Verification items for the finished model (mm, model axes). Face numbers are marked on the shaded views. A direction names the side the tool comes from. Coordinates: 2 decimals unless noted, no trailing zeros. Write each loop counter-clockwise with the first axis right and the second up, starting at its lowest first coordinate (ties: lowest second). Pieces come first, ordered by that corner, then holes. Notation, with made-up numbers: M 22,-33 L 59,-33 A32 cw 59,-2 Z; hole C 65.5,39 d2. An arc over 180 degrees is marked long. Answer in a Markdown table with one row per item.
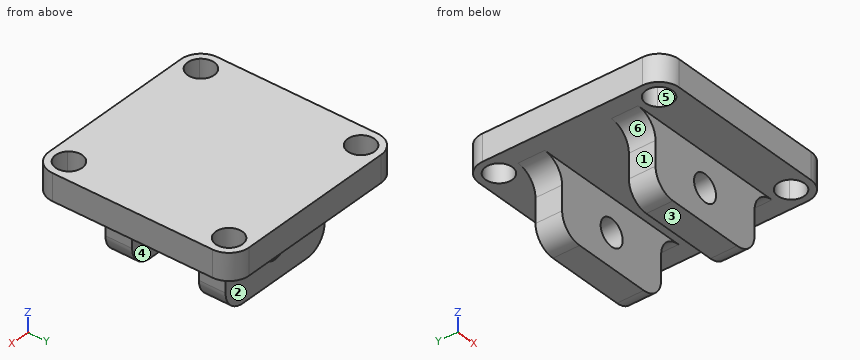
Autodesk Inventor part; units mm, degrees
ref_plane "YZ Plane" through (0, 0, 0) normal (1, 0, 0) x (0, 1, 0)
ref_plane "XZ Plane" through (0, 0, 0) normal (0, 1, 0) x (-1, 0, 0)
ref_plane "XY Plane" through (0, 0, 0) normal (0, 0, 1) x (1, 0, 0)
ref_plane "Work Plane1" through (-192, 24, -212) normal (0, 0, -1) x (-1, 0, 0)
sketch "Sketch1" plane through (-192, 24, -212) normal (0, 0, -1) x (-1, 0, 0)
  circle A0 centre (-32, -8) radius 2
  arc A1 (-30.5858, -33.4142) -> (-33.4142, -30.5858) centre (-32, -32) ccw
  arc A2 (-6.5858, -33.4142) -> (-9.4142, -30.5858) centre (-8, -32) ccw
  circle A3 centre (-8, -8) radius 2
  circle A4 centre (-32, -32) radius 2
  circle A5 centre (-8, -32) radius 2
  circle A6 centre (-8, -8) radius 2
  circle A7 centre (-32, -8) radius 2
  circle A8 centre (-32, -8) radius 3
  circle A9 centre (-8, -8) radius 3
  circle A10 centre (-8, -32) radius 3
  circle A11 centre (-32, -32) radius 3
  line L0 (-35, -8) -> (-35, -32)
  line L1 (-32, -35) -> (-8, -35)
  line L2 (-5, -32) -> (-5, -8)
  line L3 (-8, -5) -> (-32, -5)
  point P0 (-192, -24)
  point P1 (-9.4142, -30.5858)
  point P2 (-33.4142, -30.5858)
  dimension "d0" = 1
  dimension "d1" = 1
  dimension "d2" = 1
  dimension "d3" = 1
extrude "Extrusion1" add sketch "Sketch1" along normal blind 4
sketch "Sketch2" plane through (-192, 24, -216) normal (0, 0, -1) x (-1, 0, 0)
  line L0 (-35, -8) -> (-35, -32)
  line L1 (-5, -32) -> (-5, -8)
  line L2 (-5, -32) -> (-5, -8)
  line L3 (-35, -11) -> (-5, -11)
  line L4 (-5, -11) -> (-5, -29)
  line L5 (-5, -29) -> (-35, -29)
  line L6 (-35, -29) -> (-35, -11)
  circle A0 centre (-32, -8) radius 2
  circle A1 centre (-8, -8) radius 2
  circle A2 centre (-8, -32) radius 2
  circle A3 centre (-32, -32) radius 2
  line L7 (-29, -11) -> (-29, -29)
  line L8 (-11, -11) -> (-11, -29)
  point P0 (-192, -24)
  dimension "d6" = 3
  dimension "d7" = 3
  dimension "d8" = 3
  dimension "d9" = 3
extrude "Extrusion2" add sketch "Sketch2" along normal blind 10 contours L3 L8 L5 L7
sketch "Sketch3" plane through (-181, -5, -216) normal (-1, 0, 0) x (0, 0, 1)
  line L0 (0, 18) -> (0, 0)
  line L1 (0, 18) -> (-10, 18)
  line L2 (-10, 0) -> (-10, 18)
  line L3 (0, 0) -> (-10, 0)
  line L4 (-10, 18) -> (-10, 0)
  line L5 (0, 21) -> (0, -3)
  line L6 (-10, 14) -> (0, 14)
  line L7 (0, 14) -> (0, 4)
  line L8 (0, 4) -> (-10, 4)
  line L9 (-10, 4) -> (-10, 14)
  point P0 (216, 5)
  point P1 (-10, 4)
  point P2 (0, 4)
  point P3 (0, 14)
  dimension "d12" = 4
  dimension "d13" = 4
extrude "Extrusion3" cut sketch "Sketch3" against normal through all contours L0 L8 L2 L6
fillet "Fillet1" radius 3.175 8 edges at (-181, 11, -226) (-163, 11, -226) (-181, 11, -216) (-163, 11, -216) (-163, -3, -216) (-163, -3, -226) (-181, -3, -226) (-181, -3, -216)
sketch "Sketch4" plane through (-184.175, 13, -216) normal (0, 1, 0) x (1, 0, 0)
  arc A0 (21.175, 6.825) -> (18, 10) centre (18, 6.825) ccw
  line L0 (6.35, 10) -> (18, 10)
  arc A1 (6.35, 10) -> (3.175, 6.825) centre (6.35, 6.825) ccw
  line L1 (3.175, 3.175) -> (3.175, 6.825)
  arc A2 (0, 0) -> (3.175, 3.175) centre (0, 3.175) ccw
  line L2 (24.35, 0) -> (0, 0)
  arc A3 (21.175, 3.175) -> (24.35, 0) centre (24.35, 3.175) ccw
  line L3 (21.175, 3.175) -> (21.175, 6.825)
  circle A4 centre (12.175, 5) radius 2
  point P0 (184.175, -216)
  dimension "d17" = 4
  dimension "d18" = 18
  dimension "d19" = 9
  dimension "d20" = 10
  dimension "d21" = 5
extrude "Extrusion4" cut sketch "Sketch4" against normal through all contours A4
equation "\"d19\" = 0.5 * d18"
equation "\"d21\" = 0.5 * d20"
properties part number "hinge"
1) Sectioned sample at C-C (z = -224.25). Record the cut outline in (x, y), then the cut area to 3 significant figures.
Response values:
| item | result |
|---|---|
| outline | M -180.66,-5 L -163.34,-5 L -163.34,-1 L -180.66,-1 Z; M -180.66,9 L -163.34,9 L -163.34,13 L -180.66,13 Z |
| area | 139 mm² |
2) Tool access check on the marked faces 1, 2 and 3. Record the directions out of +Z, -Z, +X, -X, +Y, -Y that give a thin tool (end or side, any length) a straight path to the whole face; none if there is none.
Response values:
| item | result |
|---|---|
| face 1 | -Z, -X, +Y, -Y |
| face 2 | -Z, +X, -X, +Y |
| face 3 | -Z, +X, -X, +Y, -Y |
3) Release check for a two-part mould opening along X. For the marked faces 4, 5 and 6 record: +X half, -X half, draft (parallel to the pull), parting line (faces both ways), or undercut.
Response values:
| item | result |
|---|---|
| face 4 | draft |
| face 5 | undercut |
| face 6 | -X half |
4) Sectioned sample at B-B (y = -3.5). Record the cut outline in (x, z) (3 decimals).
Response values:
| item | result |
|---|---|
| outline | M -187,-216 L -184.175,-216 A3.175 cw -181,-219.175 L -181,-222.825 A3.175 ccw -177.825,-226 L -166.175,-226 A3.175 ccw -163,-222.825 L -163,-219.175 A3.175 cw -159.825,-216 L -157,-216 L -157,-212 L -187,-212 Z; hole C -172,-221 d4 |
5) Sectioned sample at D-D (z = -221.5). Record the cut outline in (x, y), then the cut area to 3 significant figures.
Response values:
| item | result |
|---|---|
| outline | M -181,-5 L -173.94,-5 L -173.94,-1 L -181,-1 Z; M -181,9 L -173.94,9 L -173.94,13 L -181,13 Z; M -170.06,-5 L -163,-5 L -163,-1 L -170.06,-1 Z; M -170.06,9 L -163,9 L -163,13 L -170.06,13 Z |
| area | 113 mm² |
6) Thickness scan on L1, parallel to Y at x = -184, z = -214.4; L2, parallel to Y at x = -169, z = -217; L3, parallel to Z at x = -172, y = -1.9. Record the ranges inside material, lowest first. Write a range as [from, to].
Response values:
| item | result |
|---|---|
| L1 | y = [-11, -10], [-6, 14], [18, 19] |
| L2 | y = [-5, -1], [9, 13] |
| L3 | z = [-226, -223], [-219, -212] |
7) Depth check by flat-ended pin: pin 1 (8 mm diameter, centred on x = -179, z = -223.5, fed in from -Y); pin 2 (3 mm diameter, centred on y = 11, z = -221.5, fed in from -X); pin 3 (1 mm diameter, centred on y = 10, z = -218, fed in from +X). Enter the tip coordinate at first touch or a pass-through.
Response values:
| item | result |
|---|---|
| pin 1 | stops at y = -5 |
| pin 2 | stops at x = -181 |
| pin 3 | stops at x = -162.52 |
8) Sectioned sample at A-A (x = -172). Record the cut outline in (y, z).
Response values:
| item | result |
|---|---|
| outline | M -11,-216 L -5,-216 L -5,-219 L -1,-219 L -1,-216 L 9,-216 L 9,-219 L 13,-219 L 13,-216 L 19,-216 L 19,-212 L -11,-212 Z; M -5,-226 L -1,-226 L -1,-223 L -5,-223 Z; M 9,-226 L 13,-226 L 13,-223 L 9,-223 Z |
